Check sheet for the modelled part. Datum: model origin and axes. Units: mm. Round coordinates to 2 decimals unless told otherwise and drop trailing zeros. Loops run counter-clockwise (first coordinate to the right, second up) from the corner with the lowest first, then second, coordinate; pieces in that order, holes last. Notation, with made-up numbers: (80.5, -17) - (134.5, -17) arc R8 cw to (134.5, -8) - close; hole circle Ø6 at (77, 36). An arc over 180 degrees is marked (long way). Put each result on its own line as item: value.
```python
from build123d import *

# Parameters (mm, degrees)
SKETCH1_R           = 3.175
BOSS_EXTRUDE1_DEPTH = 1.5875
FILLET1_R           = 3.175
FILLET2_R           = 1.5875


with BuildPart() as part:
    # Sketch1 → Boss-Extrude1 (new body)
    with BuildSketch(Plane(origin=(0, 0, 0), x_dir=(1, 0, 0), z_dir=(0, 1, 0))):
        with BuildLine():
            Line((-17.348522628, 0), (12.7, 0))
            Line((12.7, 0), (12.7, 1.5875))
            Line((12.7, 1.5875), (38.1, 1.5875))
            Line((38.1, 1.5875), (38.1, 61.9125))
            Line((38.1, 61.9125), (28.575, 61.9125))
            Line((28.575, 61.9125), (28.575, 11.1125))
            Line((28.575, 11.1125), (12.7, 11.1125))
            Line((12.7, 11.1125), (12.7, 12.7))
            Line((12.7, 12.7), (-17.348522628, 12.7))
            ThreePointArc((-17.348522628, 12.7), (-19.05, 6.35), (-17.348522628, 0))
        make_face()
        with Locations(Location((-6.35, 6.35, 0), (0, 0, 270))):
            Circle(SKETCH1_R, mode=Mode.SUBTRACT)
    extrude(amount=BOSS_EXTRUDE1_DEPTH)

    # Fillet1
    fillet1_edges = [part.edges().sort_by_distance(p)[0] for p in [
        (28.575, 0.79375, -11.1125),
        (28.575, 0.79375, -61.9125),
        (38.1, 0.79375, -61.9125),
        (38.1, 0.79375, -1.5875),
    ]]
    fillet(fillet1_edges, radius=FILLET1_R)

    # Fillet2
    fillet2_edges = [part.edges().sort_by_distance(p)[0] for p in [
        (12.7, 0.79375, 0),
        (12.7, 0.79375, -12.7),
    ]]
    fillet(fillet2_edges, radius=FILLET2_R - 0.0001)  # a hair under: the kernel refuses the full size


solid = part.part
```
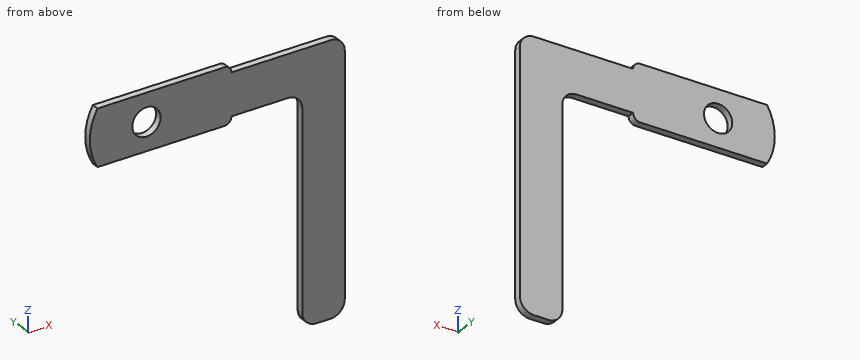
Item 1: Thickness scan on line 1 (X direction, y = 1.2, z = -6.35) (3 decimals); line 2 (Z direction, x = 8.5, y = 1.4); line 3 (X direction, y = 1.4, z = -29.5) (3 decimals). Record the ranges inside material, lowest first. Write a range as from..to.
Filled sheet:
line 1: -19.05..-9.525, -3.175..38.1
line 2: -12.7..0
line 3: 28.575..38.1
Item 2: Section check B-B on x = -6.35. Enter the section's corners in (y, z) (1 decimal).
Filled sheet:
outline: (0, -12.7) - (1.6, -12.7) - (1.6, -9.5) - (0, -9.5) - close; (0, -3.2) - (1.6, -3.2) - (1.6, 0) - (0, 0) - close
Item 3: Section check D-D on x = 23. Enter the section's corners in (y, z).
Filled sheet:
outline: (0, -11.11) - (1.59, -11.11) - (1.59, -1.59) - (0, -1.59) - close
Item 4: Go/stop test with flat-tipped pins: pin 1 (0.8 mm diameter, centred on x = 27, y = 0.5, fed in from +Z); pin 2 (0.5 mm diameter, centred on x = -5.5, y = 1, fed in from -Z). Record where each tip stops, or that it passes through.
Filled sheet:
pin 1: z = -1.59
pin 2: z = -12.7
